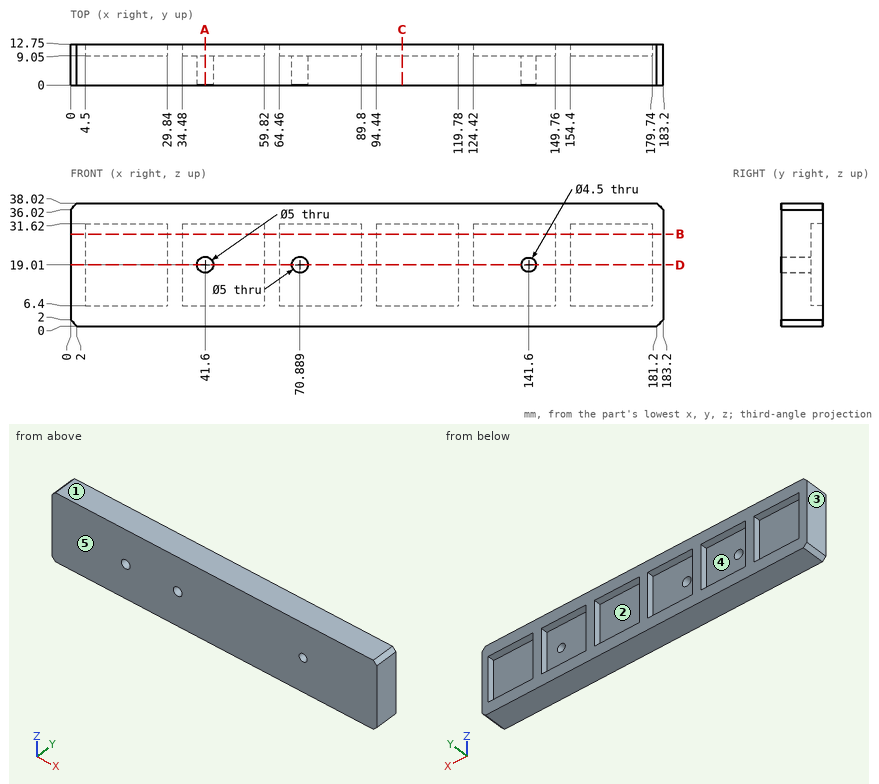
Geometry: see drawing. Coordinates: mm, zero at the bounding-box minimum. A direction names the side the tool comes from. Give positions to 0.01 mm unless a question says otherwise; leave off trailing zeros. Order: outer loops, then holes, each group sorted by start corner. A loop starts at its lowest first (then second) coordinate and runs counter-clockwise, first axis right, second up. Notation, with made-up numbers: (-30.75, 0.25) - (23.25, 0.25) arc R25 cw to (23.25, 36.25) - close; hole circle Ø5 at (-25.75, 44.5). An arc over 180 degrees is marked (long way). One line per item, written item: value.
1. Pin query (flat end, axial travel): pin 1 Ø12.5 at (x, z) = (11, 19) entering from +Y. Return the tip coordinate at first contact, or that it passes through.
Determined:
pin 1: y = 9.05
2. Cut plane A-A, the plane x = 41.6. Output: boundary loops of the cut face in (y, z), and give its area (3 significant figures).
Determined:
outline: (0, 0) - (12.75, 0) - (12.75, 6.4) - (9.05, 6.4) - (9.05, 16.51) - (0, 16.51) - close; (0, 21.51) - (9.05, 21.51) - (9.05, 31.62) - (12.75, 31.62) - (12.75, 38.02) - (0, 38.02) - close
area: 346 mm2
3. Reachability of the marked faces 4 and 5 from +Z, -Z, +X, -X, +Y, -Y: full face, straight path, thin tool, end or side. Return the list, or none.
Determined:
face 4: +Y
face 5: +Z, -Z, +X, -X, -Y
4. Line query: probe 1 along X at (y, z) = (8.75, 19); probe 2 along Z at (x, y) = (115.5, 11.75); probe 3 along Z at (x, y) = (141.6, 5.25). Output: solid intervals per line, ascending.
Determined:
probe 1: 0 to 39.1, 44.1 to 68.39, 73.39 to 139.35, 143.85 to 183.2
probe 2: 0 to 6.4, 31.62 to 38.02
probe 3: 0 to 16.76, 21.26 to 38.02
5. Cut plane C-C, the plane x = 102.5. Output: boundary loops of the cut face in (y, z).
Determined:
outline: (0, 0) - (12.75, 0) - (12.75, 6.4) - (9.05, 6.4) - (9.05, 31.62) - (12.75, 31.62) - (12.75, 38.02) - (0, 38.02) - close
6. Cut plane B-B, the plane z = 28.5. Output: boundary loops of the cut face in (x, y).
Determined:
outline: (0, 0) - (183.2, 0) - (183.2, 12.75) - (179.74, 12.75) - (179.74, 9.05) - (154.4, 9.05) - (154.4, 12.75) - (149.76, 12.75) - (149.76, 9.05) - (124.42, 9.05) - (124.42, 12.75) - (119.78, 12.75) - (119.78, 9.05) - (94.44, 9.05) - (94.44, 12.75) - (89.8, 12.75) - (89.8, 9.05) - (64.46, 9.05) - (64.46, 12.75) - (59.82, 12.75) - (59.82, 9.05) - (34.48, 9.05) - (34.48, 12.75) - (29.84, 12.75) - (29.84, 9.05) - (4.5, 9.05) - (4.5, 12.75) - (0, 12.75) - close
7. Cut plane D-D, the plane z = 19.01. Give the number of separate pieces and of enclosed holes in the cut face, and give its area (3 significant figures).
Determined:
separate pieces: 4
enclosed holes: 0
area: 1,640 mm2
8. Draft query along X for the marked faces 1, 2 and 3. Return one class per face: released by +X, released by -X, zero draft, split by the parting line, or undercut.
Determined:
face 1: zero draft
face 2: undercut
face 3: released by -X
